Solid Edge part; units mm, degrees
sketch "Sketch1" plane through (0, 0, 0) normal (0, 0, 1) x (1, 0, 0)
  circle A0 centre (0, 0) radius 145
extrude "Protrusion1" add sketch "Sketch1" along normal blind 12
hole "Bohrung_1" at (-20, 0, 12) direction (0, 0, -1) diameter 4.917 depth 10 thread major 6 thread length 8
hole "Hole1" at (20, 0, 12) direction (0, 0, -1) diameter 4.917 depth 10 thread major 6 thread length 8
hole "Bohrung_3" at (-110, 42.5, 12) direction (0, 0, -1) diameter 4.917 depth 10 thread major 6 thread length 8
hole "Hole2" at (-110, 27.5, 12) direction (0, 0, -1) diameter 4.917 depth 10 thread major 6 thread length 8
hole "Bohrung_9" at (42.5, -110, 12) direction (0, 0, -1) diameter 4.917 depth 10 thread major 6 thread length 8
hole "Hole3" at (27.5, -110, 12) direction (0, 0, -1) diameter 4.917 depth 10 thread major 6 thread length 8
hole "Bohrung_11" at (48, -48, 12) direction (0, 0, -1) diameter 8.376 depth 9 thread major 10 thread length 8
hole "Hole4" at (-48, -48, 12) direction (0, 0, -1) diameter 8.376 depth 9 thread major 10 thread length 8
hole "Hole5" at (-48, 48, 12) direction (0, 0, -1) diameter 8.376 depth 9 thread major 10 thread length 8
hole "Hole6" at (48, 48, 12) direction (0, 0, -1) diameter 8.376 depth 9 thread major 10 thread length 8
Input: part model. Units: mm. Frame: model coordinates. A direction names the side the tool comes from. Round coordinates to 2 decimals unless told otherwise and drop trailing zeros. Write each loop counter-clockwise with the first axis right and the second up, starting at its lowest first coordinate (ties: lowest second). Pieces come first, ordered by that corner, then holes.
1) Cut plane C-C (x = 77). Return the cut outline in (y, z), then the cut area to 3 significant figures.
2) Reachability of faces 4 (the flat face through (-2, 2, 0)), 5 (the flat face through (-48, 48, 3)) from +Z, -Z, +X, -X, +Y, -Y: full face, straight path, thin tool, end or side. Return the list, or none.
3) Contact query for flat-ended pins moving along their axis: P1, Ø4.5, axis at x = -110, y = 27.5, coming from the -Z side; P2, Ø6, axis at y = -57.5, z = 3, coming from the -X side; P3, Ø4, axis at x = -47, y = 49.5, coming from the +Z side; P4, Ø4.5, axis at x = 42.5, y = -110, coming from the +Z side. Output: stop coordinate, or through.
4) Cut plane A-A (z = 7.5). Count the separate pieces of the cut face and the enclosed holes in it, then the cut area to 3 significant figures.
5) Draft query along Y for faces 1 (the flat face through (-2, 2, 12)), 2 (the cylindrical face through (-46.4, -51.87, 7.44)), 3 (the cylindrical face through (138.304, -43.554, 5.916)). Return one class per face: pulls with the +Y half, pulls with the -Y half, needs draft (parallel to the pull), parting line crosses it, or undercut.
6) Ray query, L1, parallel to X at y = -110, z = 9; L2, parallel to X at y = -48, z = 5; L3, parallel to Y at x = 42.5, z = 6.75. Return the intervals inside material, ascending.
7) Cut plane D-D (x = -40). Return the cut outline in (y, z).
8) Cut plane B-B (y = -48). Return the cut outline in (x, z), then the cut area to 3 significant figures.
Geometry says:
1. outline: (-122.87, 0) - (122.87, 0) - (122.87, 12) - (-122.87, 12) - close
1. area: 2,950 mm2
2. face 4: -Z, +X, -X, +Y, -Y
2. face 5: +Z
3. P1: stops at z = 0
3. P2: stops at x = -134.37
3. P3: stops at z = 3
3. P4: stops at z = 2
4. separate pieces: 1
4. enclosed holes: 10
4. area: 65,700 mm2
5. face 1: needs draft
5. face 2: undercut
5. face 3: parting line crosses it
6. L1: x = -94.47 to 25.04, 29.96 to 40.04, 44.96 to 94.47
6. L2: x = -136.82 to -52.19, -43.81 to 43.81, 52.19 to 136.82
6. L3: y = -138.63 to -112.46, -107.54 to 138.63
7. outline: (-139.37, 0) - (139.37, 0) - (139.37, 12) - (-139.37, 12) - close
8. outline: (-136.82, 0) - (136.82, 0) - (136.82, 12) - (52.19, 12) - (52.19, 3) - (43.81, 3) - (43.81, 12) - (-43.81, 12) - (-43.81, 3) - (-52.19, 3) - (-52.19, 12) - (-136.82, 12) - close
8. area: 3,130 mm2
